from build123d import *

# Parameters (mm, degrees)
SKETCH_1_R               = 20
SKETCH_1_R_2             = 15
EXTRUDE_1_DEPTH          = 6
CHAMFER_1_SIZE           = 1
CUT_EXTRUDE_1_DEPTH      = 10
PATTERN_CIRCULAR_1_COUNT = 4


with BuildPart() as part:
    # 草图1 → 凸台-拉伸1 (new body)
    with BuildSketch(Plane(origin=(0, 0, 0), x_dir=(0, 0, -1), z_dir=(1, 0, 0))):
        Circle(SKETCH_1_R)
        Circle(SKETCH_1_R_2, mode=Mode.SUBTRACT)
    extrude(amount=EXTRUDE_1_DEPTH)

    # 倒角1
    chamfer_1_edges = [part.edges().sort_by_distance(p)[0] for p in [
        (6, 0, 20),
        (0, 0, 20),
    ]]
    chamfer(chamfer_1_edges, length=CHAMFER_1_SIZE)

    # 草图2 → 切除-拉伸1 (cut)
    with BuildSketch(Plane(origin=(6, 0, 0), x_dir=(0, 0, -1), z_dir=(1, 0, 0))):
        with BuildLine():
            Line((16.958588854, -1.185860054), (20.747478718, -1.450805043))
            ThreePointArc((20.747478718, -1.450805043), (20.798141947, 0), (20.747478718, 1.450805043))
            Line((20.747478718, 1.450805043), (16.958588854, 1.185860054))
            ThreePointArc((16.958588854, 1.185860054), (17, 0), (16.958588854, -1.185860054))
        make_face()
    cut_extrude_1 = extrude(amount=-CUT_EXTRUDE_1_DEPTH, mode=Mode.SUBTRACT)

    # 阵列(圆周)1: 切除-拉伸1 ×4 about axis
    pattern_circular_1_axis = Axis((6, 0, 0), (1, 0, 0))
    for i in range(1, PATTERN_CIRCULAR_1_COUNT):
        add(cut_extrude_1.rotate(pattern_circular_1_axis, i * 360 / PATTERN_CIRCULAR_1_COUNT), mode=Mode.SUBTRACT)


solid = part.part
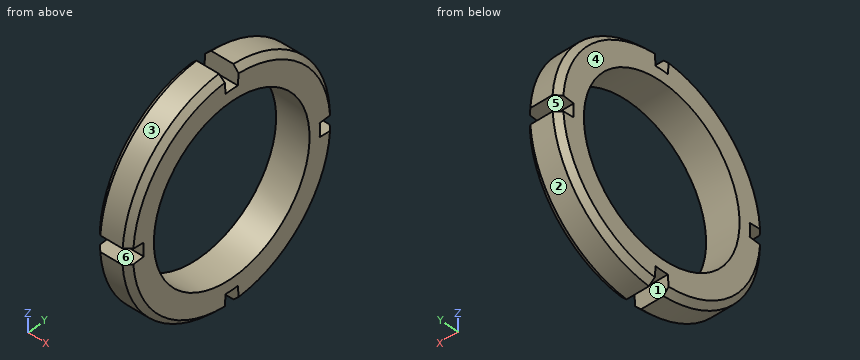
Can you work these out from the model? Positions are in its coordinate system, mm. Face numbers are marked on the shaded views. A direction names the side the tool comes from. Coordinates: 2 decimals unless noted, no trailing zeros. Loops run counter-clockwise (first coordinate to the right, second up) from the corner with the lowest first, then second, coordinate; pieces in that order, holes last. Notation, with made-up numbers: M -0.75,11.5 L 39.25,11.5 A9 ccw 39.25,19.5 Z; hole C 65,-29.5 d9. An arc over 180 degrees is marked long. Return JSON: item names as keys, results as strings. Group by question number.
Item 1: On a 3-axis mill with a long thin cutter (end or side, diameter ignored), from which of +Z, -Z, +X, -X, +Y, -Y can I reach the whole of each face in a straight line? I mean the marked faces 4, 5 and 6. Say none if no direction works.
Item 2: If I drill on L1, parallel to Y at x = 3.1, z = 0; L2, parallel to Z at x = 4.5, y = 5.5; L3, parallel to Z at x = 1.25, y = -1, over which ranges is the centre line in solid material (lowest first)? Write a range as from..to.
Item 3: Imagine slicing it at A-A (z = 0). Please give me the cut outline in (x, y).
Item 4: I'm going to push flat-ended pins straight in: pin 1 Ø1 at (x, z) = (0.5, 0.5) entering from -Y; pin 2 Ø2 at (x, y) = (1, 13) entering from -Z. Where does each tip first touch, or does it pass through?
Item 5: Thinking about a two-plate mould opening in Y: for the marked faces 1, 2 and 3, which applies, released by +Y, released by -Y, zero draft, split by the parting line, or undercut?
Item 6: Imagine slicing it at C-C (x = 0.5). Please give me the cut outline in (y, z), and give its area (3 significant figures).
Verdict:
{
 "1": {"face 4": "+Z, -Z, -X, +Y, -Y", "face 5": "+X, -X, +Y", "face 6": "+X, -X, -Y"},
 "2": {"L1": "y = -17..-15, 15..17", "L2": "z = -19.23..-13.96, 13.96..19.23", "L3": "z = -16.97..-14.97, 14.97..16.97"},
 "3": {"outline": "M 0,-17 L 6,-17 L 6,-15 L 0,-15 Z; M 0,15 L 6,15 L 6,17 L 0,17 Z"},
 "4": {"pin 1": "stops at y = -17", "pin 2": "stops at z = -16"},
 "5": {"face 1": "undercut", "face 2": "released by +Y", "face 3": "released by -Y"},
 "6": {"outline": "M -19.45,-1.36 A19.5 ccw -1.36,-19.45 L -1.19,-16.96 A17 ccw 1.19,-16.96 L 1.36,-19.45 A19.5 ccw 19.45,-1.36 L 16.96,-1.19 A17 ccw 16.96,1.19 L 19.45,1.36 A19.5 ccw 1.36,19.45 L 1.19,16.96 A17 ccw -1.19,16.96 L -1.36,19.45 A19.5 ccw -19.45,1.36 L -16.96,1.19 A17 ccw -16.96,-1.19 Z; hole C 0,0 d30", "area": "462 mm^2"}
}
